For this review, use the dimensioned drawing (mm, ordinates from the lowest corner) and the shaded views. A direction names the side the tool comes from. Coordinates: 2 decimals unless noted, no trailing zeros. Loops run counter-clockwise (first coordinate to the right, second up) from the corner with the lowest first, then second, coordinate; pieces in that order, holes last.
1. To check wall thickness, follow probe 1 along Y at (x, z) = (28.5, 22.85); probe 2 along Y at (x, z) = (43.5, 21.75) (1 decimal); probe 3 along X at (y, z) = (11.5, 20.75) (1 decimal). State the ranges of each line that lie inside material, in increasing order.
2. Take a section at B-B, the plane x = 52.5. State the section outline as (y, z) points, then the cut area to 3 significant figures.
3. Clearance check with flat-ended pins moving along their axes: P1, Ø8, axis at x = 23.5, z = 9, coming from the -Y side; P2, Ø2, axis at y = 15.5, z = 16.5, coming from the +X side; P3, Ø1.5, axis at y = 40.5, z = 7.5, coming from the -X side. State where each tip first meets the part, or that it passes through.
4. Take a section at A-A, the plane y = 28.5. State the section outline as (x, z) points.
5. Machinability: for the marked faces 5 and 6, which of the approach directions +Z, -Z, +X, -X, +Y, -Y give a long, thin tool a straight path to every point of the face, cutting with its end or side? Answer none if there is none.
6. Take a section at C-C, the plane x = 28.5. State the section outline as (y, z) points.
7. Mouldability with a two-part tool opening along Z and no side actions: class the marked faces 1, 2, 3 and 4 as pulls with the +Z half, pulls with the -Z half, needs draft (parallel to the pull), parting line crosses it, or undercut.
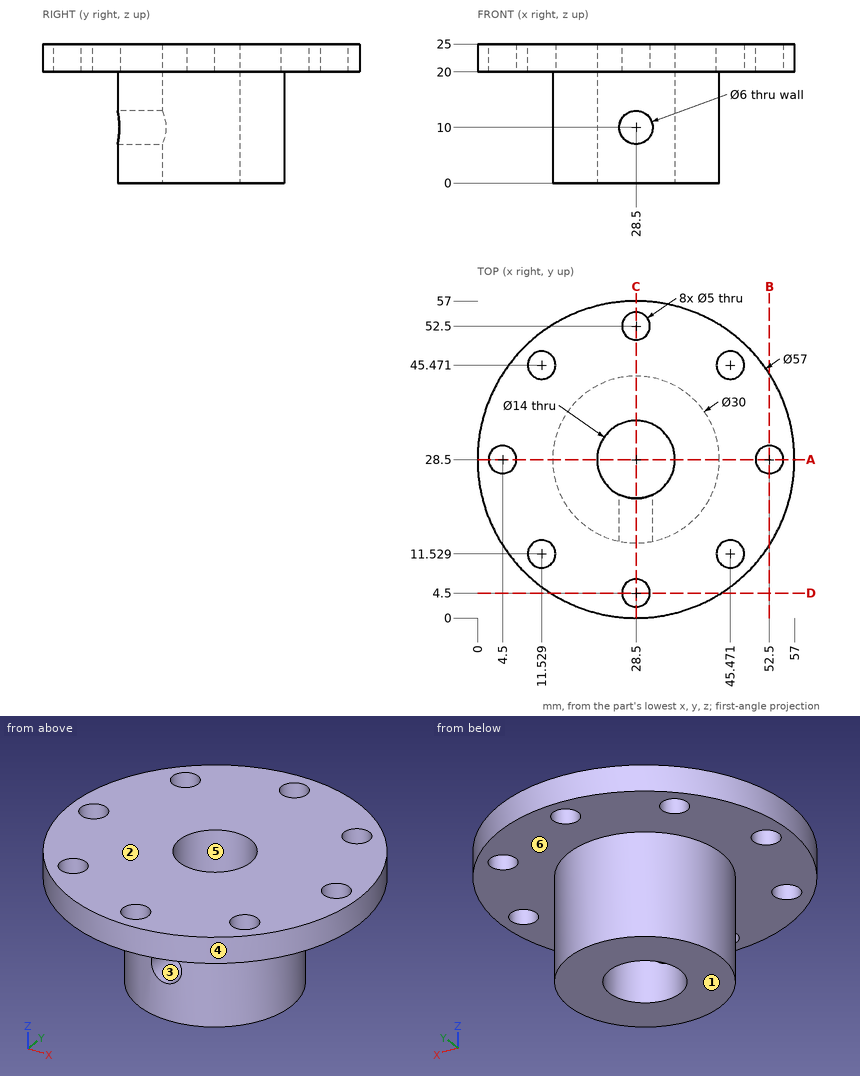
Results list:
1. probe 1: y = 0 to 2, 7 to 21.5, 35.5 to 50, 55 to 57
1. probe 2: y = 4.3 to 10, 13.1 to 43.9, 47 to 52.7
1. probe 3: x = 5.6 to 9, 14 to 43, 48 to 51.4
2. outline: (13.13, 20) - (26, 20) - (26, 25) - (13.13, 25) - close; (31, 20) - (43.87, 20) - (43.87, 25) - (31, 25) - close
2. area: 129 mm2
3. P1: stops at y = 13.56
3. P2: stops at x = 37.5
3. P3: stops at x = 18.58
4. outline: (0, 20) - (2, 20) - (2, 25) - (0, 25) - close; (7, 20) - (13.5, 20) - (13.5, 0) - (21.5, 0) - (21.5, 25) - (7, 25) - close; (35.5, 0) - (43.5, 0) - (43.5, 20) - (50, 20) - (50, 25) - (35.5, 25) - close; (55, 20) - (57, 20) - (57, 25) - (55, 25) - close
5. face 5: +Z, -Z
5. face 6: -Z
6. outline: (0, 20) - (2, 20) - (2, 25) - (0, 25) - close; (7, 20) - (13.5, 20) - (13.5, 13) - (21.5, 13) - (21.5, 25) - (7, 25) - close; (13.5, 0) - (21.5, 0) - (21.5, 7) - (13.5, 7) - close; (35.5, 0) - (43.5, 0) - (43.5, 20) - (50, 20) - (50, 25) - (35.5, 25) - close; (55, 20) - (57, 20) - (57, 25) - (55, 25) - close
7. face 1: pulls with the -Z half
7. face 2: pulls with the +Z half
7. face 3: undercut
7. face 4: needs draft
